```python
from build123d import *

# Parameters (mm, degrees)
SKETCH1_R            = 15
BOSS_EXTRUDE1_DEPTH  = 5
SKETCH2_R            = 15
SKETCH2_R_2          = 10
BOSS_EXTRUDE2_DEPTH  = 27
SKETCH4_R            = 3
BOSS_EXTRUDE19_DEPTH = 16
BOSS_EXTRUDE20_DEPTH = 6
LPATTERN1_COUNT      = 2
LPATTERN1_PITCH      = 112
BOSS_EXTRUDE21_START = -6
BOSS_EXTRUDE21_DEPTH = 6
BOSS_EXTRUDE22_START = 24
SKETCH8_R            = 2.5
SKETCH8_R_2          = 15
BOSS_EXTRUDE22_DEPTH = 6
BOSS_EXTRUDE23_DEPTH = 7
BOSS_EXTRUDE24_DEPTH = 2


with BuildPart() as part:
    # Sketch1 → Boss-Extrude1 (new body)
    with BuildSketch(Plane(origin=(0, 0, 0), x_dir=(1, 0, 0), z_dir=(0, 1, 0))):
        with BuildLine():
            Line((-18, 48.505826631), (-18, 14.317821063))
            ThreePointArc((-18, 14.317821063), (-23, 0), (-18, -14.317821063))
            Line((-18, -14.317821063), (-18, -48.505826631))
            Line((-18, -48.505826631), (-39.526711514, -64.145898034))
            ThreePointArc((-39.526711514, -64.145898034), (-41.706339098, -70.854101966), (-36, -75))
            Line((-36, -75), (36, -75))
            ThreePointArc((36, -75), (41.706339098, -70.854101966), (39.526711514, -64.145898034))
            Line((39.526711514, -64.145898034), (18, -48.505826631))
            Line((18, -48.505826631), (18, -14.317821063))
            ThreePointArc((18, -14.317821063), (23, 0), (18, 14.317821063))
            Line((18, 14.317821063), (18, 48.505826631))
            Line((18, 48.505826631), (39.526711514, 64.145898034))
            ThreePointArc((39.526711514, 64.145898034), (41.706339098, 70.854101966), (36, 75))
            Line((36, 75), (-36, 75))
            ThreePointArc((-36, 75), (-41.706339098, 70.854101966), (-39.526711514, 64.145898034))
            Line((-39.526711514, 64.145898034), (-18, 48.505826631))
        make_face()
        with Locations(Location((0, 0, 0), (0, 0, 270))):
            Circle(SKETCH1_R, mode=Mode.SUBTRACT)
    extrude(amount=BOSS_EXTRUDE1_DEPTH)



with BuildPart() as body_2:
    # Sketch2 → Boss-Extrude2 (new body)
    with BuildSketch(Plane.XY.offset(75)):
        with Locations((0, 67)):
            Circle(SKETCH2_R)
        with Locations((0, 67)):
            Circle(SKETCH2_R_2, mode=Mode.SUBTRACT)
    extrude(amount=-BOSS_EXTRUDE2_DEPTH)


with BuildPart() as part_1:
    add(part.part)

    add(body_2.part)  # Boss-Extrude19 merges body 2
    # Sketch4 → Boss-Extrude19 (add)
    with BuildSketch(Plane.XY.offset(75)):
        with BuildLine():
            Line((-6, 53.252272915), (-6, 31))
            Line((-6, 31), (-11, 31))
            ThreePointArc((-11, 31), (-18, 24), (-11, 17))
            Line((-11, 17), (-6, 17))
            Line((-6, 17), (-6, 5))
            Line((-6, 5), (6, 5))
            Line((6, 5), (6, 17))
            Line((6, 17), (11, 17))
            ThreePointArc((11, 17), (18, 24), (11, 31))
            Line((11, 31), (6, 31))
            Line((6, 31), (6, 53.252272915))
            ThreePointArc((6, 53.252272915), (0, 52), (-6, 53.252272915))
        make_face()
        with Locations((-11, 24)):
            Circle(SKETCH4_R, mode=Mode.SUBTRACT)
        with Locations((11, 24)):
            Circle(SKETCH4_R, mode=Mode.SUBTRACT)
    extrude(amount=-BOSS_EXTRUDE19_DEPTH)

    # Sketch5 → Boss-Extrude20 (add)
    with BuildSketch(Plane(origin=(0, 0, 59), x_dir=(-1, 0, 0), z_dir=(0, 0, -1))):
        with BuildLine():
            Line((-20, 5), (-20, 49))
            Line((-20, 49), (-10.723697691, 56.511801497))
            ThreePointArc((-10.723697691, 56.511801497), (0, 52), (10.723697691, 56.511801497))
            Line((10.723697691, 56.511801497), (20, 49))
            Line((20, 49), (20, 5))
            Line((20, 5), (-20, 5))
        make_face()
    boss_extrude20 = extrude(amount=BOSS_EXTRUDE20_DEPTH)

    # LPattern1: Boss-Extrude20 ×2
    with Locations(*[(0, 0, -i * LPATTERN1_PITCH) for i in range(1, LPATTERN1_COUNT)]):
        add(boss_extrude20)

    # Sketch7 → Boss-Extrude21 (add)
    with BuildSketch(Plane(origin=(0, 0, -59), x_dir=(-1, 0, 0), z_dir=(0, 0, -1)).offset(BOSS_EXTRUDE21_START)):
        with BuildLine():
            Line((-10.723697691, 56.511801497), (10.723697691, 56.511801497))
            ThreePointArc((10.723697691, 56.511801497), (0, 52), (-10.723697691, 56.511801497))
        make_face()
    extrude(amount=BOSS_EXTRUDE21_DEPTH)

    # Sketch8 → Boss-Extrude22 (add)
    with BuildSketch(Plane(origin=(0, 5, 0), x_dir=(1, 0, 0), z_dir=(0, 1, 0)).offset(BOSS_EXTRUDE22_START)):
        with BuildLine():
            Line((-36.150207697, 5.601482559), (-18, 12.568694522))
            Line((-18, 12.568694522), (-18, 53))
            Line((-18, 53), (18, 53))
            Line((18, 53), (18, 12.568694522))
            Line((18, 12.568694522), (36.150207697, 5.601482559))
            ThreePointArc((36.150207697, 5.601482559), (40, 0), (36.150207697, -5.601482559))
            Line((36.150207697, -5.601482559), (18, -12.568694522))
            Line((18, -12.568694522), (18, -53))
            Line((18, -53), (15, -53))
            Line((15, -53), (15, -48))
            Line((15, -48), (-15, -48))
            Line((-15, -48), (-15, -53))
            Line((-15, -53), (-18, -53))
            Line((-18, -53), (-18, -12.568694522))
            Line((-18, -12.568694522), (-36.150207697, -5.601482559))
            ThreePointArc((-36.150207697, -5.601482559), (-40, 0), (-36.150207697, 5.601482559))
        make_face()
        with Locations(Location((-34, 0, 0), (0, 0, 270))):
            Circle(SKETCH8_R, mode=Mode.SUBTRACT)
        with Locations(Location((34, 0, 0), (0, 0, 270))):
            Circle(SKETCH8_R, mode=Mode.SUBTRACT)
        with Locations(Location((0, 0, 0), (0, 0, 270))):
            Circle(SKETCH8_R_2, mode=Mode.SUBTRACT)
    extrude(amount=BOSS_EXTRUDE22_DEPTH)

    # Sketch9 → Boss-Extrude23 (add, symmetric)
    with BuildSketch(Plane(origin=(0, 0, 0), x_dir=(0, 0, -1), z_dir=(1, 0, 0))):
        with BuildLine():
            Line((53, 51.511801497), (32.799551055, 51.511801497))
            ThreePointArc((32.799551055, 51.511801497), (29.799551055, 50.997082871), (27.142696805, 49.511801497))
            ThreePointArc((27.142696805, 49.511801497), (23.626903958, 49.884897539), (24, 53.400690386))
            ThreePointArc((24, 53.400690386), (28.132884388, 55.711128079), (32.799551055, 56.511801497))
            Line((32.799551055, 56.511801497), (53, 56.511801497))
            Line((53, 56.511801497), (53, 51.511801497))
        make_face()
    extrude(amount=BOSS_EXTRUDE23_DEPTH, both=True)

    # Sketch10 → Boss-Extrude24 (add, symmetric)
    with BuildSketch(Plane(origin=(0, 0, 0), x_dir=(0, 0, -1), z_dir=(1, 0, 0))):
        with BuildLine():
            Line((75, 5), (64.145898034, 5))
            Line((64.145898034, 5), (59, 5))
            Line((59, 5), (59, 49))
            Line((59, 49), (59, 56.511801497))
            Line((59, 56.511801497), (53, 56.511801497))
            Line((53, 56.511801497), (32.799551055, 56.511801497))
            ThreePointArc((32.799551055, 56.511801497), (31.5778479, 56.458393963), (30.365465911, 56.29857884))
            Line((30.365465911, 56.29857884), (59, 61.35406732))
            ThreePointArc((59, 61.35406732), (63.46156073, 60.365729702), (65.917079571, 56.511801497))
            Line((65.917079571, 56.511801497), (75, 5))
        make_face()
    extrude(amount=BOSS_EXTRUDE24_DEPTH, both=True)


solid = part_1.part
```
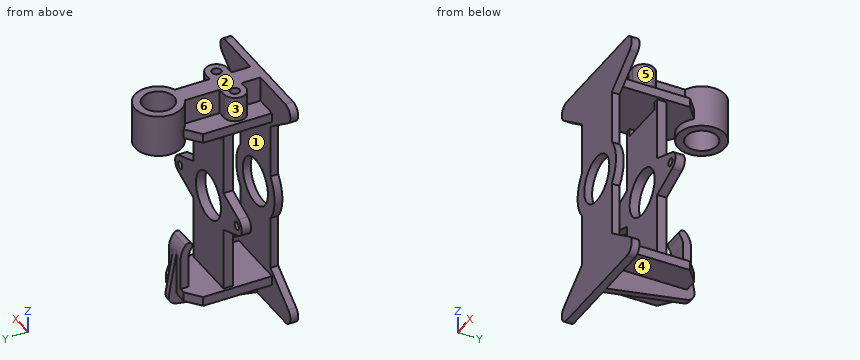
CAD build for the part. Positions are in the model's coordinates, mm. Face numbers are marked on the shaded views. A direction names the side the tool comes from. Give positions to 0.01 mm unless a question says otherwise; leave off trailing zeros. Loops run counter-clockwise (first coordinate to the right, second up) from the corner with the lowest first, then second, coordinate; pieces in that order, holes last. Notation, with made-up numbers: (57, 32) - (98, 32) arc R13 ccw to (98, 49) - close; hole circle Ø7 at (-26, 23.5). An arc over 180 degrees is marked (long way). Put each result on its own line as item: value.
Q1. Slice it at D-D (z = -36). Give the cut face in (x, y).
Filled in:
outline: (-18, 0) - (18, 0) - (18, 5) - (-18, 5) - close; (-18, 29) - (18, 29) - (18, 35) - (-18, 35) - close; (-7, 51.51) - (7, 51.51) - (7, 56.51) - (2, 56.51) - (2, 57.29) - (-2, 57.29) - (-2, 56.51) - (-7, 56.51) - close
Q2. Mould opens along Z. For the marked faces 1, 2 and 3 say: pulls with the +Z half, pulls with the -Z half, needs draft (parallel to the pull), parting line crosses it, or undercut.
Filled in:
face 1: undercut
face 2: pulls with the +Z half
face 3: needs draft
Q3. Probe line 1 along X through (y, z) = (30.75, 0); line 2 along X through (y, z) = (3.5, 0); line 3 along Y through (x, z) = (11.5, -48.5). List the from-to ranges inside material, lowest first.
Filled in:
line 1: x = -40 to -36.5, -31.5 to -15, 15 to 31.5, 36.5 to 40
line 2: x = -23 to -15, 15 to 23
line 3: y = 0 to 5, 29 to 35
Q4. Slice it at A-A (y = 67). Give the cut face in (x, z).
Filled in:
outline: (-15, 48) - (-10, 48) - (-10, 75) - (-15, 75) - close; (10, 48) - (15, 48) - (15, 75) - (10, 75) - close
Q5. Tool access for the marked faces 4, 5 and 6: list every direction of +Z, -Z, +X, -X, +Y, -Y with a clear straight run to the whole face (end or side of a thin tool).
Filled in:
face 4: -Z, +X, +Y
face 5: +Z, +X
face 6: +Z, -X
Q6. Slice it at C-C (z = 0). Give the cut face in (x, y), plus the area to 3 significant figures.
Filled in:
outline: (-40, 29) - (-36.5, 29) - (-36.5, 35) - (-40, 35) - close; (-31.5, 29) - (-15, 29) - (-15, 35) - (-31.5, 35) - close; (-23, 0) - (-15, 0) - (-15, 5) - (-23, 5) - close; (15, 0) - (23, 0) - (23, 5) - (15, 5) - close; (15, 29) - (31.5, 29) - (31.5, 35) - (15, 35) - close; (36.5, 29) - (40, 29) - (40, 35) - (36.5, 35) - close
area: 320 mm²
Q7. Slice it at B-B (x = 0). Give the number of separate pieces and of enclosed holes in the cut face, plus the area to 3 significant figures.
Filled in:
separate pieces: 4
enclosed holes: 0
area: 3,470 mm²
Q8. Flat gauge pins, fed straight in: pin 1 (6.5 mm diameter, centred on y = 33.5, z = -41.5, fed in from +X); pin 2 (5 mm diameter, centred on y = 38.5, z = 69.5, fed in from -X); pin 3 (12 mm diameter, centred on x = -15.5, z = 7, fed in from +Y). Where does each tip first touch, or does it go through?
Filled in:
pin 1: stops at x = 18
pin 2: stops at x = -6
pin 3: stops at y = 35
